Verification items for the finished model (mm, model axes). Round coordinates to 2 decimals unless told otherwise and drop trailing zeros. Loops run counter-clockwise (first coordinate to the right, second up) from the corner with the lowest first, then second, coordinate; pieces in that order, holes last. Notation, with made-up numbers: (-24, 19) -> (16, 19) arc R14 ccw to (16, 31) -> close; hole circle Ø1 at (62.25, -31). An arc over 180 degrees is marked (long way). Write item = value, one per line.
```python
from build123d import *

# Parameters (mm, degrees)
SKETCH1_W           = 490
SKETCH1_H           = 106.02
BOSS_EXTRUDE1_DEPTH = 6
SKETCH2_W           = 6
SKETCH2_H           = 24
CUT_EXTRUDE1_DEPTH  = 502.374351558
SKETCH3_W           = 157.333333333
SKETCH3_H           = 6
CUT_EXTRUDE2_DEPTH  = 502.374351558


with BuildPart() as part:
    # Sketch1 → Boss-Extrude1 (new body)
    with BuildSketch(Plane.XY):
        with Locations((245, 53.01)):
            Rectangle(SKETCH1_W, SKETCH1_H)
    extrude(amount=BOSS_EXTRUDE1_DEPTH)

    # Sketch2 → Cut-Extrude1 (cut, through all)
    with BuildSketch(Plane.XY.offset(6)):
        with Locations((487, 12)):
            Rectangle(SKETCH2_W, SKETCH2_H)
        with Locations((487, 94.02)):
            Rectangle(SKETCH2_W, SKETCH2_H)
        with Locations((3, 94.02)):
            Rectangle(SKETCH2_W, SKETCH2_H)
        with Locations((3, 12)):
            Rectangle(SKETCH2_W, SKETCH2_H)
    extrude(amount=-CUT_EXTRUDE1_DEPTH, mode=Mode.SUBTRACT)

    # Sketch3 → Cut-Extrude2 (cut, through all)
    with BuildSketch(Plane.XY.offset(6)):
        with Locations((84.666666667, 3)):
            Rectangle(SKETCH3_W, SKETCH3_H)
        with Locations((405.333333334, 3)):
            Rectangle(SKETCH3_W, SKETCH3_H)
        with Locations((84.666666667, 103.02)):
            Rectangle(SKETCH3_W, SKETCH3_H)
        with Locations((405.333333334, 103.02)):
            Rectangle(SKETCH3_W, SKETCH3_H)
    extrude(amount=-CUT_EXTRUDE2_DEPTH, mode=Mode.SUBTRACT)


solid = part.part
```
(1) Go/stop test with flat-tipped pins: pin 1 Ø3 at (y, z) = (22, 5) entering from -X; pin 2 Ø1.8 at (x, z) = (2, 2) entering from +Y; pin 3 Ø1.8 at (y, z) = (3.5, 3.5) entering from +X. Record where each tip stops, or that it passes through.
Filled sheet:
pin_1 = 6
pin_2 = 82.02
pin_3 = 326.67
(2) Sectioned sample at B-B, the plane x = 44. Record the cut outline in (y, z).
Filled sheet:
outline = (6, 0) -> (100.02, 0) -> (100.02, 6) -> (6, 6) -> close
(3) Sectioned sample at A-A, the plane z = 3.1. Record the cut outline in (x, y).
Filled sheet:
outline = (0, 24) -> (6, 24) -> (6, 6) -> (163.33, 6) -> (163.33, 0) -> (326.67, 0) -> (326.67, 6) -> (484, 6) -> (484, 24) -> (490, 24) -> (490, 82.02) -> (484, 82.02) -> (484, 100.02) -> (326.67, 100.02) -> (326.67, 106.02) -> (163.33, 106.02) -> (163.33, 100.02) -> (6, 100.02) -> (6, 82.02) -> (0, 82.02) -> close
(4) Material ranges on probe 1 along Y at (x, z) = (340.5, 2.05); probe 2 along X at (y, z) = (11, 5.75), recorded low to high. Write a range as from..to.
Filled sheet:
probe_1 = 6..100.02
probe_2 = 6..484
